The model under review builds one solid part; all positions refer to its coordinate system, in mm. Face numbers are marked on the shaded views. A direction names the side the tool comes from. Round coordinates to 2 decimals unless told otherwise and drop trailing zeros. Write each loop counter-clockwise with the first axis right and the second up, starting at its lowest first coordinate (ties: lowest second). Pieces come first, ordered by that corner, then holes. Notation, with made-up numbers: (49.5, 59) -> (78.5, 59) arc R34 ccw to (78.5, 89) -> close; hole circle Ø6 at (67.5, 50). An arc over 180 degrees is marked (long way). Answer as a JSON object with one key per item and string values. Group by question number.
1) Mouldability with a two-part tool opening along X and no side actions: class the marked faces 5, 6 and 7 as pulls with the +X half, pulls with the -X half, needs draft (parallel to the pull), parting line crosses it, or undercut.
2) We need section B-B, the plane z = -7. Write out the cut boundary in (x, y).
3) To check wall thickness, follow probe 1 along Y at (x, z) = (16.5, -0.5). State the ranges of the line that lie inside material, in increasing order. Write a range as [from, to].
4) We need section C-C, the plane y = -11. Write out the cut boundary in (x, z), then the cut area to 3 significant figures.
5) Insertion check: pin 1 Ø1.5 at (y, z) = (6.5, -1) entering from -X. The pin has a flat end and moves straight along its axis. Give the tip position at first contact, or say it passes through.
6) We need section A-A, the plane x = -7. Write out the cut boundary in (y, z).
7) Machinability: for the marked faces 1, 2, 3 and 4, which of the approach directions +Z, -Z, +X, -X, +Y, -Y give a long, thin tool a straight path to every point of the face, cutting with its end or side? Answer none if there is none.
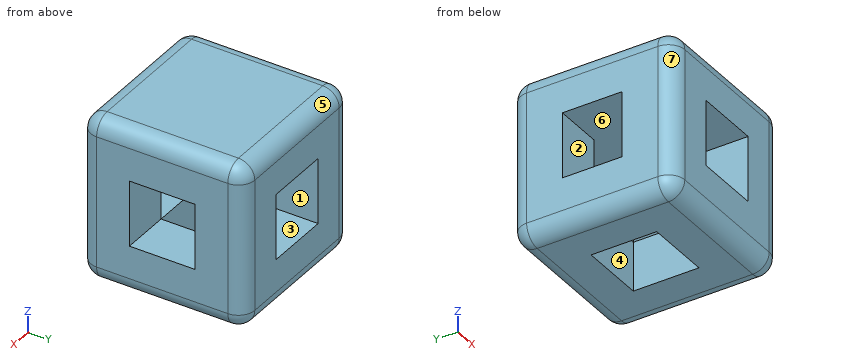
from build123d import *

# Parameters (mm, degrees)
F0_W      = 50
F0_H      = 50
F1_DEPTH  = 25
F2_W      = 20
F2_H      = 20
F3_DEPTH  = 50
F4_W      = 20
F4_H      = 20
F5_DEPTH  = 15
F6_W      = 18.1838367134
F6_H      = 20
F7_DEPTH  = 15
F8_R      = 5
F9_W      = 20
F9_H      = 20
F10_DEPTH = 15


with BuildPart() as f1:
    # F0 (on Front) → F1 (new body, symmetric)
    with BuildSketch(Plane.XZ):
        Rectangle(F0_W, F0_H)
    extrude(amount=F1_DEPTH, both=True)

    # F2 (on face) → F3 (cut, through all)
    with BuildSketch(Plane.XZ.offset(25)):
        Rectangle(F2_W, F2_H)
    extrude(amount=-F3_DEPTH, mode=Mode.SUBTRACT)

    # F4 (on face) → F5 (cut, through all)
    with BuildSketch(Plane.YZ.offset(25)):
        Rectangle(F4_W, F4_H)
    extrude(amount=-F5_DEPTH, mode=Mode.SUBTRACT)

    # F6 (on face) → F7 (cut, through all)
    with BuildSketch(Plane(origin=(-25, 0, 0), x_dir=(0, -1, 0), z_dir=(-1, 0, 0))):
        Rectangle(F6_W, F6_H)
    extrude(amount=-F7_DEPTH, mode=Mode.SUBTRACT)

    # F8
    f8_edges = [f1.edges().sort_by_distance(p)[0] for p in [
        (0, -25, -25),
        (25, 0, -25),
        (0, 25, -25),
        (-25, 0, -25),
        (-25, -25, 0),
        (-25, 25, 0),
        (-25, 0, 25),
        (25, 0, 25),
        (0, 25, 25),
        (0, -25, 25),
        (25, -25, 0),
        (25, 25, 0),
    ]]
    fillet(f8_edges, radius=F8_R)

    # F9 (on face) → F10 (cut, through all)
    with BuildSketch(Plane(origin=(0, 0, -25), x_dir=(1, 0, 0), z_dir=(0, 0, -1))):
        Rectangle(F9_W, F9_H)
    extrude(amount=-F10_DEPTH, mode=Mode.SUBTRACT)


solid = f1.part
Here are the results:
{
 "1": {"face 5": "needs draft", "face 6": "undercut", "face 7": "pulls with the -X half"},
 "2": {"outline": "(-25, -20) arc R5 ccw to (-20, -25) -> (-10, -25) -> (-10, -9.09) -> (-25, -9.09) -> close; (-25, 9.09) -> (-10, 9.09) -> (-10, 25) -> (-20, 25) arc R5 ccw to (-25, 20) -> close; (10, -25) -> (20, -25) arc R5 ccw to (25, -20) -> (25, -10) -> (10, -10) -> close; (10, 10) -> (25, 10) -> (25, 20) arc R5 ccw to (20, 25) -> (10, 25) -> close"},
 "3": {"probe 1": "y = [-25, -10], [10, 25]"},
 "4": {"outline": "(-25, -20) arc R5 ccw to (-20, -25) -> (20, -25) arc R5 ccw to (25, -20) -> (25, 20) arc R5 ccw to (20, 25) -> (-20, 25) arc R5 ccw to (-25, 20) -> close; hole (-10, -10) -> (10, -10) -> (10, 10) -> (-10, 10) -> close", "area": "2,080 mm^2"},
 "5": {"pin 1": "passes through"},
 "6": {"outline": "(-25, -20) arc R5 ccw to (-20, -25) -> (-10, -25) -> (-10, -10) -> (-25, -10) -> close; (-25, 10) -> (25, 10) -> (25, 20) arc R5 ccw to (20, 25) -> (-20, 25) arc R5 ccw to (-25, 20) -> close; (10, -25) -> (20, -25) arc R5 ccw to (25, -20) -> (25, -10) -> (10, -10) -> close"},
 "7": {"face 1": "none", "face 2": "+X, -X", "face 3": "+Y, -Y", "face 4": "-Z"}
}
